Autodesk Inventor part; units mm, degrees
ref_plane "Work Plane1" through (29, 0, 0) normal (0, -1, 0) x (1, 0, 0)
ref_plane "YZ Plane" through (0, 0, 0) normal (1, 0, 0) x (0, 1, 0)
ref_plane "XZ Plane" through (0, 0, 0) normal (0, 1, 0) x (-1, 0, 0)
sketch "Sketch1" plane through (0, 0, 0) normal (0, 0, 1) x (1, 0, 0)
  line L0 (-0.0667, 0) -> (8, 0)
  line L1 (8, 0) -> (8, 2)
  line L2 (8, 2) -> (2.1, 2)
  line L3 (2.1, 2) -> (1.6705, 2)
  line L4 (1.6705, 2) -> (0, 2)
  line L5 (0, 2) -> (0, 3.8)
  line L6 (0, 3.8) -> (-2.2, 3.8)
  line L7 (-2.2, 3.8) -> (-2.2, 1.4434)
  line L8 (-2.2, 1.4434) -> (-0.9, 1.4434)
  line L9 (-0.9, 1.4434) -> (-0.0667, 0)
  line L10 (-4.24, 0) -> (10.04, 0)
  line L11 (0, -0.76) -> (0, 4.56)
  line L12 (2.1, 2) -> (0, 2) construction
  dimension "d1" = 5.9
  dimension "d2" = 0.4295
  dimension "d3" = 2.2
  dimension "d4" = 1.3
  dimension "d5" = 60
  dimension "d6" = 4
  dimension "d7" = 4
  dimension "d8" = 2.8868
  dimension "d9" = 7.6
  dimension "d26" = 8
revolve "Body" add sketch "Sketch1" angle 360 about axis through (-0.0667, 0, 0) along (1, 0, 0)
sketch "Sketch2" plane through (-2.2, 0, 0) normal (-1, 0, 0) x (0, 0, 1)
  circle A0 centre (0, 0) radius 1.4434
  line L0 (0, -5.32) -> (0, 5.32)
  line L1 (-5.32, 0) -> (5.32, 0)
  line L2 (1.4434, 0) -> (0.7217, -1.25)
  line L3 (0.7217, -1.25) -> (-0.7217, -1.25)
  line L4 (-0.7217, -1.25) -> (-1.4434, 0)
  line L5 (-1.4434, 0) -> (-0.7217, 1.25)
  line L6 (-0.7217, 1.25) -> (0.7217, 1.25)
  line L7 (0.7217, 1.25) -> (1.4434, 0)
  point P0 (0, 0)
extrude "Slot" add sketch "Sketch2" against normal up to next contours L7 A0 | A0 L2 | L6 L0 A0 | A0 L0 L3 | L0 L6 A0 | A0 L3 L0 | L4 A0 | A0 L5
fillet "Fillet1" radius 1.9 1 edges at (-2.2, -3.8, 0)
thread "Thread"
chamfer "Chamfer1" distance 0.4294 distance2 0.4294 1 edges at (8, -2, 0) measured on face at (8, 0.556, 0.0273)
ref_plane "Work Plane1" through (29, 0, 0) normal (0, -1, 0) x (1, 0, 0)
fillet "Fillet2" radius 0.4 1 edges at (0, -2, 0)
equation "\"d1\" = GEL"
equation "\"d3\" = KOH"
equation "\"d4\" = INTI"
equation "\"d6\" = GD"
equation "\"d7\" = BDM"
equation "\"d8\" = 1.1547 * SW"
equation "\"d9\" = KOD"
equation "\"d26\" = NLG"
equation "\"d30\" = R"
equation "\"d17\" = RR"
equation "\"d13\" = GEL"
equation "\"d15\" = -0.5 * SPD + 0.5 * GD"
equation "\"d16\" = GUL"
equation "\"GD\" = NND"
equation "\"NLG\" = 8"
equation "\"GEL\" = 5.9"
equation "\"KOD\" = 7.6"
equation "\"KOH\" = 2.2"
equation "\"INTI\" = 1.3"
equation "\"GAL\" = 0.61345 * PTC"
equation "\"GUL\" = 0.61345 * PTC"
equation "\"BDM\" = NND"
equation "\"SW\" = 2.5"
equation "\"RR\" = 1.9"
equation "\"SPD\" = NND - 1.2269 * PTC"
equation "\"R\" = 0.4"
equation "\"TOA\" = 30deg"
equation "\"GD1\" = THREADDIA - 1.2269 * PTC"
equation "\"THREADDIA\" = 4"
equation "\"PTC\" = 0.7"
equation "\"NND\" = 4"
equation "\"KOH1\" = 0.3"
equation "\"E0\" = 2.873"
properties part number "ISO 7380-1 - M4 x 8" material "Steel"
Work out the finished part from the listing and answer in its coordinate system (mm). A direction names the side the tool comes from. Round coordinates to 2 decimals unless told otherwise and drop trailing zeros. Write each loop counter-clockwise with the first axis right and the second up, starting at its lowest first coordinate (ties: lowest second). Pieces come first, ordered by that corner, then holes.
1) A cutting plane is placed at A-A (x = 3.5). Give the vertices of the cut face in (y, z).
2) Straight lines are drawn through the part: line 1 (Z direction, x = -1.5, y = 2.5); line 2 (Z direction, x = -1.25, y = 3.25); line 3 (X direction, y = 0, z = -1). For each, find the intervals that lie inside material, in ascending order.
3) Given pin 1 Ø4 at (x, y) = (2.5, -2) entering from -Z; pin 2 Ø1 at (x, z) = (4.5, -1.5) entering from -Y; pin 3 Ø1 at (y, z) = (2.5, -2.5) entering from +X, each flat-ended and moving along its own axis, determine where each tip first touches the part or whether it passes through.
4) A tool of negligible diameter and unlimited length cuts with its end or side. For faces 1 (the flat face through (0, 2.5, -0.8)), 2 (the cylindrical face through (-0.15, -2.8, -2.57)), 3 (the flat face through (-1.5, -0.63, -1.08)), from which of +Z, -Z, +X, -X, +Y, -Y can it reach the whole face along a straight path? Write none if from no direction.
Completed:
1. outline: circle Ø4 at (0, 0)
2. line 1: z = -2.26 to 2.26
2. line 2: z = -1.42 to 1.42
2. line 3: x = -0.64 to 8
3. pin 1: stops at z = -2
3. pin 2: stops at y = -1.73
3. pin 3: stops at x = 0
4. face 1: +X
4. face 2: +X, -X
4. face 3: -X
